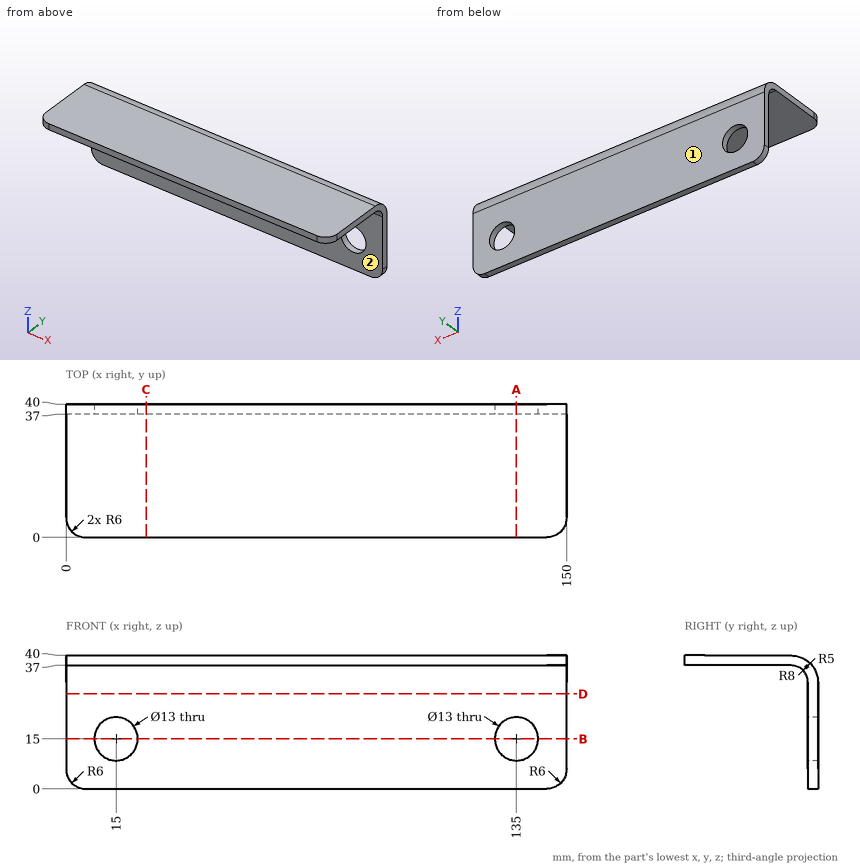
Input: dimensioned drawing with shaded views. Units: mm. Origin: part minimum x, y, z. A direction names the side the tool comes from. Round coordinates to 2 decimals unless told otherwise and drop trailing zeros. Loops run counter-clockwise (first coordinate to the right, second up) from the corner with the lowest first, then second, coordinate; pieces in that order, holes last. Notation, with made-up numbers: (45, 66.25) -> (74, 66.25) arc R32 ccw to (74, 97.25) -> close; hole circle Ø11 at (-37.75, -20). An arc over 180 degrees is marked (long way). One line per item, written item: value.
(1) Section D-D (z = 28.5). Return the cut outline in (x, y), plus the area to 3 significant figures.
Geometry check:
outline: (0, 37) -> (150, 37) -> (150, 40) -> (0, 40) -> close
area: 450 mm2
(2) Set-up query: the marked faces 1 and 2. Return all of +Z, -Z, +X, -X, +Y, -Y with unobstructed straight access to the full face (end or side cutting, diameter ignored); none if empty.
Geometry check:
face 1: +Z, -Z, +X, -X, +Y
face 2: -Z, +X, -X, -Y
(3) Section B-B (z = 15). Return the cut outline in (x, y).
Geometry check:
outline: (0, 37) -> (8.5, 37) -> (8.5, 40) -> (0, 40) -> close; (21.5, 37) -> (128.5, 37) -> (128.5, 40) -> (21.5, 40) -> close; (141.5, 37) -> (150, 37) -> (150, 40) -> (141.5, 40) -> close
(4) Section A-A (x = 135). Return the cut outline in (y, z), plus the area to 3 significant figures.
Geometry check:
outline: (0, 37) -> (32, 37) arc R5 cw to (37, 32) -> (37, 21.5) -> (40, 21.5) -> (40, 32) arc R8 ccw to (32, 40) -> (0, 40) -> close; (37, 0) -> (40, 0) -> (40, 8.5) -> (37, 8.5) -> close
area: 184 mm2
(5) Section C-C (x = 24). Return the cut outline in (y, z).
Geometry check:
outline: (0, 37) -> (32, 37) arc R5 cw to (37, 32) -> (37, 0) -> (40, 0) -> (40, 32) arc R8 ccw to (32, 40) -> (0, 40) -> close
(6) Material intervals for line 1 (Y direction, x = 7, z = 22); line 2 (Z direction, x = 15, y = 38), sorted ascending. Write a range as [from, to].
Geometry check:
line 1: [37, 40]
line 2: [0, 8.5], [21.5, 37.29]
(7) Pin query (flat end, axial travel): pin 1 (5 mm diameter, centred on x = 62, y = 10, fed in from -Z); pin 2 (1 mm diameter, centred on x = 66, y = 34, fed in from +Z); pin 3 (1 mm diameter, centred on x = 38, z = 25.5, fed in from -Y). Return the tip coordinate at first contact, or that it passes through.
Geometry check:
pin 1: z = 37
pin 2: z = 39.86
pin 3: y = 37
